from build123d import *

# Parameters (mm, degrees)
F1_DEPTH = 1955.8
F3_DEPTH = 1.27
F5_DEPTH = 1.27


with BuildPart() as f1:
    # F0 (on Right) → F1 (new body)
    with BuildSketch(Plane.YZ):
        Polygon((-152.4, 0), (0, 0), (0, 152.4), align=None)
        Polygon((-149.333949, 1.27), (-1.27, 149.333949), (-1.27, 1.27), align=None, mode=Mode.SUBTRACT)
    extrude(amount=F1_DEPTH)

    # F2 (on face) → F3 (join)
    with BuildSketch(Plane(origin=(0, 0, 0), x_dir=(0, -1, 0), z_dir=(-1, 0, 0))):
        Polygon((1.27, 149.333949), (1.27, 1.27), (149.333949, 1.27), align=None)
    extrude(amount=-F3_DEPTH)

    # F4 (on face) → F5 (join)
    with BuildSketch(Plane.YZ.offset(1955.8)):
        Polygon((-149.333949, 1.27), (-1.27, 1.27), (-1.27, 149.333949), align=None)
    extrude(amount=-F5_DEPTH)


solid = f1.part
Build history of the part. All positions in model axes, mm. A direction names the side the tool comes from. Round coordinates to 2 decimals unless told otherwise and drop trailing zeros. Write each loop counter-clockwise with the first axis right and the second up, starting at its lowest first coordinate (ties: lowest second). Pieces come first, ordered by that corner, then holes. Notation, with made-up numbers: (0.25, -29) -> (11.25, -29) arc R12 cw to (11.25, -14) -> close; hole circle Ø5 at (50, -29). An arc over 180 degrees is marked (long way). Use one line per item in the form item = value.
Q1. Two-plate mould, pull along Y, no slides. Class faces 1 (the flat face through (964, -77, 0)), 2 (the flat face through (964.2, -75.1, 77.3)), 3 (the flat face through (964.227, -76.338, 74.266)): released by +Y, released by -Y, zero draft, split by the parting line, or undercut.
Conclusion:
face_1 = zero draft
face_2 = released by -Y
face_3 = undercut
Q2. Band-saw the part on A-A, the plane z = 133. Write the cut outline in (x, y).
Conclusion:
outline = (0, -19.4) -> (1955.8, -19.4) -> (1955.8, 0) -> (0, 0) -> close; hole (1.27, -17.6) -> (1954.53, -17.6) -> (1954.53, -1.27) -> (1.27, -1.27) -> close
Q3. Band-saw the part on C-C, the plane y = -90.5. Write the cut outline in (x, z).
Conclusion:
outline = (0, 0) -> (1955.8, 0) -> (1955.8, 61.9) -> (0, 61.9) -> close; hole (1.27, 1.27) -> (1954.53, 1.27) -> (1954.53, 60.1) -> (1.27, 60.1) -> close
Q4. Drill centre lines: L1, parallel to X at y = -17, z = 31.5; L2, parallel to Z at x = 111, y = -33; L3, parallel to Y at x = 196, z = 136.5. Where is each one in solid material? Low to high.
Conclusion:
L1 = 0 to 1.27, 1954.53 to 1955.8
L2 = 0 to 1.27, 117.6 to 119.4
L3 = -15.9 to -14.1, -1.27 to 0
Q5. Tool access for faces 4 (the flat face through (0, -41, 43)), 5 (the flat face through (964, -74, 1.27)): list every direction of +Z, -Z, +X, -X, +Y, -Y with a clear straight run to the whole face (end or side of a thin tool).
Conclusion:
face_4 = +Z, -Z, -X, +Y, -Y
face_5 = none
Q6. Drop flat-ended pins along their axis: P1, Ø2, axis at x = 579.5, z = 23.5, coming from the -Y side; P2, Ø3, axis at x = 1346, y = -120.5, coming from the +Z side; P3, Ø6, axis at x = 476.5, z = 128, coming from the -Y side. Give the stop position or say it passes through.
Conclusion:
P1 = -129.9
P2 = 33.4
P3 = -27.4
Q7. Band-saw the part on B-B, the plane x = 856. Write the cut outline in (y, z).
Conclusion:
outline = (-152.4, 0) -> (0, 0) -> (0, 152.4) -> close; hole (-149.33, 1.27) -> (-1.27, 1.27) -> (-1.27, 149.33) -> close
